Build history of the part. All positions in model axes, mm. Give positions to 0.01 mm unless a question says otherwise; leave off trailing zeros. Order: outer loops, then holes, each group sorted by start corner. A loop starts at its lowest first (then second) coordinate and runs counter-clockwise, first axis right, second up. Notation, with made-up numbers: M 60.25,79 L 96.25,79 A22 cw 96.25,118 Z; hole C -8,74.25 d3. An arc over 180 degrees is marked long. One line per item, written item: value.
from build123d import *

# Parameters (mm, degrees)
SKETCH1_W            = 498.348
SKETCH1_H            = 165.1
BOSS_EXTRUDE1_DEPTH  = 1.5875
BOSS_EXTRUDE2_DEPTH  = 3.175
CUT_EXTRUDE1_DEPTH   = 3.175
LPATTERN1_COUNT      = 5
LPATTERN1_PITCH      = 88.9
SKETCH4_R            = 3.675
CUT_EXTRUDE2_DEPTH   = 4.175
LPATTERN2_COUNT      = 2
LPATTERN2_PITCH      = 38.1
SKETCH5_W            = 3.175
SKETCH5_H            = 88.9
CUT_EXTRUDE3_DEPTH   = 4.175
SKETCH6_W            = 2.286
SKETCH6_H            = 107.442
CUT_EXTRUDE4_DEPTH   = 4.175
LPATTERN3_COUNT      = 4
LPATTERN3_PITCH      = 98.8568
SKETCH7_W            = 50.8
SKETCH7_H            = 3.175
BOSS_EXTRUDE3_DEPTH  = 3.175
M6_CLEARANCE_HOLE1_D = 6.6
LPATTERN4_COUNT      = 3
LPATTERN4_PITCH      = 98.8568
LPATTERN4_COL_COUNT  = 3
LPATTERN4_COL_PITCH  = 98.8568


with BuildPart() as part:
    # Sketch1 → Boss-Extrude1 (new body, symmetric)
    with BuildSketch(Plane(origin=(0, 0, 0), x_dir=(0, 0, -1), z_dir=(1, 0, 0))):
        Rectangle(SKETCH1_W, SKETCH1_H)
    extrude(amount=BOSS_EXTRUDE1_DEPTH, both=True)

    # Sketch2 → Boss-Extrude2 (add)
    with BuildSketch(Plane(origin=(1.5875, 0, 0), x_dir=(0, 0, -1), z_dir=(1, 0, 0))):
        Polygon((-249.174, -139.7), (192.024, -139.7), (249.174, -82.55), (-249.174, -82.55), align=None)
    extrude(amount=-BOSS_EXTRUDE2_DEPTH)

    # Sketch3 → Cut-Extrude1 (cut)
    with BuildSketch(Plane(origin=(1.5875, 0, 0), x_dir=(0, 0, -1), z_dir=(1, 0, 0))):
        with BuildLine():
            ThreePointArc((-222.877, -130.81), (-221.800617421, -133.408617421), (-219.202, -134.485))
            Line((-219.202, -134.485), (-219.202, -130.81))
            Line((-219.202, -130.81), (-222.877, -130.81))
        make_face()
        with BuildLine():
            Line((-219.202, -130.81), (-219.202, -134.485))
            ThreePointArc((-219.202, -134.485), (-216.603382579, -133.408617421), (-215.527, -130.81))
            ThreePointArc((-215.527, -130.81), (-219.202, -127.135), (-222.877, -130.81))
            Line((-222.877, -130.81), (-219.202, -130.81))
        make_face()
    cut_extrude1 = extrude(amount=-CUT_EXTRUDE1_DEPTH, mode=Mode.SUBTRACT)

    # LPattern1: Cut-Extrude1 ×5
    with Locations(*[(0, 0, -i * LPATTERN1_PITCH) for i in range(1, LPATTERN1_COUNT)]):
        add(cut_extrude1, mode=Mode.SUBTRACT)

    # Sketch4 → Cut-Extrude2 (cut, through all)
    with BuildSketch(Plane(origin=(1.5875, 0, 0), x_dir=(0, 0, -1), z_dir=(1, 0, 0))):
        with Locations((198.310179285, -117.249359697)):
            Circle(SKETCH4_R)
    cut_extrude2 = extrude(amount=-CUT_EXTRUDE2_DEPTH, mode=Mode.SUBTRACT)

    # LPattern2: Cut-Extrude2 ×2
    with Locations(*[Vector(0, 0.707106781, -0.707106781) * (i * LPATTERN2_PITCH) for i in range(1, LPATTERN2_COUNT)]):
        add(cut_extrude2, mode=Mode.SUBTRACT)

    # Sketch5 → Cut-Extrude3 (cut, through all)
    with BuildSketch(Plane.ZY.offset(1.5875)):
        with Locations((-247.5865, 38.1)):
            Rectangle(SKETCH5_W, SKETCH5_H)
        with Locations((247.5865, 38.1)):
            Rectangle(SKETCH5_W, SKETCH5_H)
    extrude(amount=-CUT_EXTRUDE3_DEPTH, mode=Mode.SUBTRACT)

    # Sketch6 → Cut-Extrude4 (cut, through all)
    with BuildSketch(Plane.ZY.offset(1.5875)):
        with Locations((-148.2852, 28.829)):
            Rectangle(SKETCH6_W, SKETCH6_H)
    cut_extrude4 = extrude(amount=-CUT_EXTRUDE4_DEPTH, mode=Mode.SUBTRACT)

    # LPattern3: Cut-Extrude4 ×4
    with Locations(*[(0, 0, i * LPATTERN3_PITCH) for i in range(1, LPATTERN3_COUNT)]):
        add(cut_extrude4, mode=Mode.SUBTRACT)

    # Sketch7 → Boss-Extrude3 (add)
    with BuildSketch(Plane.ZY.offset(1.5875)):
        with Locations((0, 84.1375)):
            Rectangle(SKETCH7_W, SKETCH7_H)
    extrude(amount=-BOSS_EXTRUDE3_DEPTH)

    # M6 Clearance Hole1 (through all)
    with Locations(Plane(origin=(1.5875, 0, 0), x_dir=(0, 0, -1), z_dir=(1, 0, 0))):
        with Locations((0, -73.8124)):
            m6_clearance_hole1 = Hole(M6_CLEARANCE_HOLE1_D / 2)

    # LPattern4: M6 Clearance Hole1 ×3
    with Locations(*[(0, 0, i * LPATTERN4_PITCH) for i in range(1, LPATTERN4_COUNT)]):
        add(m6_clearance_hole1, mode=Mode.SUBTRACT)

    # LPattern4 col: M6 Clearance Hole1 ×3
    with Locations(*[(0, 0, -i * LPATTERN4_COL_PITCH) for i in range(1, LPATTERN4_COL_COUNT)]):
        add(m6_clearance_hole1, mode=Mode.SUBTRACT)


solid = part.part
1) Pin check, flat tips, straight feed: pin 1 (1 mm diameter, centred on x = -0.5, y = 34.5, fed in from +Z); pin 2 (1.5 mm diameter, centred on x = 1, y = 26.5, fed in from -Z); pin 3 (0.7 mm diameter, centred on x = -0.5, z = -149, fed in from +Y). Stop position of each tip, or through.
Check values:
pin 1: z = 246
pin 2: z = -246
pin 3: y = -24.89
2) Drill centre lines: probe 1 along Z at (x, y) = (-0.7, 56.5); probe 2 along Z at (x, y) = (-0.5, -13); probe 3 along Y at (x, z) = (0.45, 0) (3 decimals). Where is each one in solid material? Low to high. Write a range as from..to.
Check values:
probe 1: -246..-149.43, -147.14..-50.57, -48.29..48.29, 50.57..147.14, 149.43..246
probe 2: -249.17..-149.43, -147.14..-50.57, -48.29..48.29, 50.57..147.14, 149.43..249.17
probe 3: -139.7..-77.112, -70.512..85.725
3) Saw through at A-A, the plane y = 60. Write the cut outline in (x, z).
Check values:
outline: M -1.59,-246 L 1.59,-246 L 1.59,-149.43 L -1.59,-149.43 Z; M -1.59,-147.14 L 1.59,-147.14 L 1.59,-50.57 L -1.59,-50.57 Z; M -1.59,-48.29 L 1.59,-48.29 L 1.59,48.29 L -1.59,48.29 Z; M -1.59,50.57 L 1.59,50.57 L 1.59,147.14 L -1.59,147.14 Z; M -1.59,149.43 L 1.59,149.43 L 1.59,246 L -1.59,246 Z
4) Saw through at B-B, the plane x = 0.1. Give the number of separate pieces and of enclosed holes in the cut face, then the cut area to 3 significant figures.
Check values:
separate pieces: 1
enclosed holes: 12
area: 107,000 mm^2
